The model under review builds one solid part; all positions refer to its coordinate system, in mm. A direction names the side the tool comes from. Coordinates: 2 decimals unless noted, no trailing zeros. Write each loop counter-clockwise with the first axis right and the second up, starting at its lowest first coordinate (ties: lowest second). Pieces come first, ordered by that corner, then holes. Notation, with made-up numbers: M -7.75,56 L 9.25,56 A34 ccw 9.25,91 Z; hole C 0,29.25 d4. An arc over 180 degrees is marked long. Answer as a JSON object with one key per item and string values.
```python
from build123d import *

# Parameters (mm, degrees)
SKETCH2_R          = 1.2573
CUT_EXTRUDE1_DEPTH = 3.175


with BuildPart() as part:
    # Sketch1 → Revolve1 (revolve)
    with BuildSketch(Plane.XY, mode=Mode.PRIVATE) as revolve1_sk:
        Polygon((0, 40.7), (3.45, 40.7), (3.45, 33.7), (3.95, 33.7), (3.95, 26.7), (12.827467985, 26.7), (13.95, 25.577467985), (13.95, 2.6), (3, 2.6), (3, 0), (0, 0), align=None)
    revolve(revolve1_sk.sketch.rotate(Axis((0, 0, 0), (0, 1, 0)), 90), axis=Axis((0, 0, 0), (0, 1, 0)))

    # Sketch2 → Cut-Extrude1 (cut)
    with BuildSketch(Plane.XZ.offset(-2.6)):
        with Locations(Location((-9.5, 0, 0), (0, 0, 270))):
            Circle(SKETCH2_R)
        with Locations(Location((0, -8, 0), (0, 0, 270))):
            Circle(SKETCH2_R)
        with Locations(Location((9.5, 0, 0), (0, 0, 270))):
            Circle(SKETCH2_R)
        with Locations(Location((0, 8, 0), (0, 0, 270))):
            Circle(SKETCH2_R)
    extrude(amount=-CUT_EXTRUDE1_DEPTH, mode=Mode.SUBTRACT)


solid = part.part
```
(1) For pin 1 Ø0.8 at (x, z) = (-0.5, 7.5) entering from -Y (3 decimals); pin 2 Ø3 at (x, z) = (0, -8) entering from -Y; pin 3 Ø2 at (x, z) = (0, 8) entering from +Y, all flat-tipped, find the tip position at first contact; note any pin that passes through.
Results list:
{"pin 1": "y = 5.775", "pin 2": "y = 2.6", "pin 3": "y = 26.7"}
(2) Add section B-B on y = 38.5. Give the boundary of the cut face in (x, z).
Results list:
{"outline": "C 0,0 d6.9"}
(3) Add section C-C on y = 28.5. Give the boundary of the cut face in (x, z), and give its area (3 significant figures).
Results list:
{"outline": "C 0,0 d7.9", "area": "49.0 mm²"}
(4) Draft analysis for pull direction Z (two halves, no side actions). For faces 1 (the face through (-0.2, 2.6, 3.3)), 2 (the face through (-2.67, 30.15, 2.91)), 3 (the face through (10, 5.775, 0)), state which applies: released by +Z, released by -Z, zero draft, split by the parting line, or undercut.
Results list:
{"face 1": "zero draft", "face 2": "split by the parting line", "face 3": "undercut"}
(5) Wall thickness on line 1 along X through (y, z) = (4, 0); line 2 along Y through (x, z) = (4.25, -1.25); line 3 along Z through (x, y) = (10.75, 23.5): over which ranges is each line inside the solid? List them lowest first. Write a range as from..to.
Results list:
{"line 1": "-13.95..-10.76, -8.24..8.24, 10.76..13.95", "line 2": "2.6..26.7", "line 3": "-8.89..8.89"}
(6) For faces 4 (the face through (-2.332, 37.151, 2.543)), 5 (the face through (0, 0, 0)), 6 (the face through (-8.253, 4.165, 0.164)), list the 3-axis set-ups (+Z, -Z, +X, -X, +Y, -Y) from which the entire face can be reached by the end or side of a thin tool; tool diameter is ignored.
Results list:
{"face 4": "+Y", "face 5": "+Z, -Z, +X, -X, -Y", "face 6": "-Y"}
(7) Add section A-A on x = 0. Give the boundary of the cut face in (y, z) (3 decimals).
Results list:
{"outline": "M 0,-3 L 2.6,-3 L 2.6,-6.743 L 5.775,-6.743 L 5.775,-9.257 L 2.6,-9.257 L 2.6,-13.95 L 25.577,-13.95 L 26.7,-12.827 L 26.7,-3.95 L 33.7,-3.95 L 33.7,-3.45 L 40.7,-3.45 L 40.7,3.45 L 33.7,3.45 L 33.7,3.95 L 26.7,3.95 L 26.7,12.827 L 25.577,13.95 L 2.6,13.95 L 2.6,9.257 L 5.775,9.257 L 5.775,6.743 L 2.6,6.743 L 2.6,3 L 0,3 Z"}
